Check sheet for the drawn part. Datum: minimum x, y, z corner. Units: mm. Coordinates: 2 decimals unless noted, no trailing zeros. Order: outer loops, then holes, each group sorted by start corner. A loop starts at its lowest first (then second) coordinate and runs counter-clockwise, first axis right, second up. Notation, with made-up numbers: (0.5, 41.5) -> (21.5, 41.5) arc R14 cw to (21.5, 47.5) -> close; hole circle Ø6 at (-14, -5). An arc over 180 degrees is marked (long way). Answer as CSV lines item,"result".
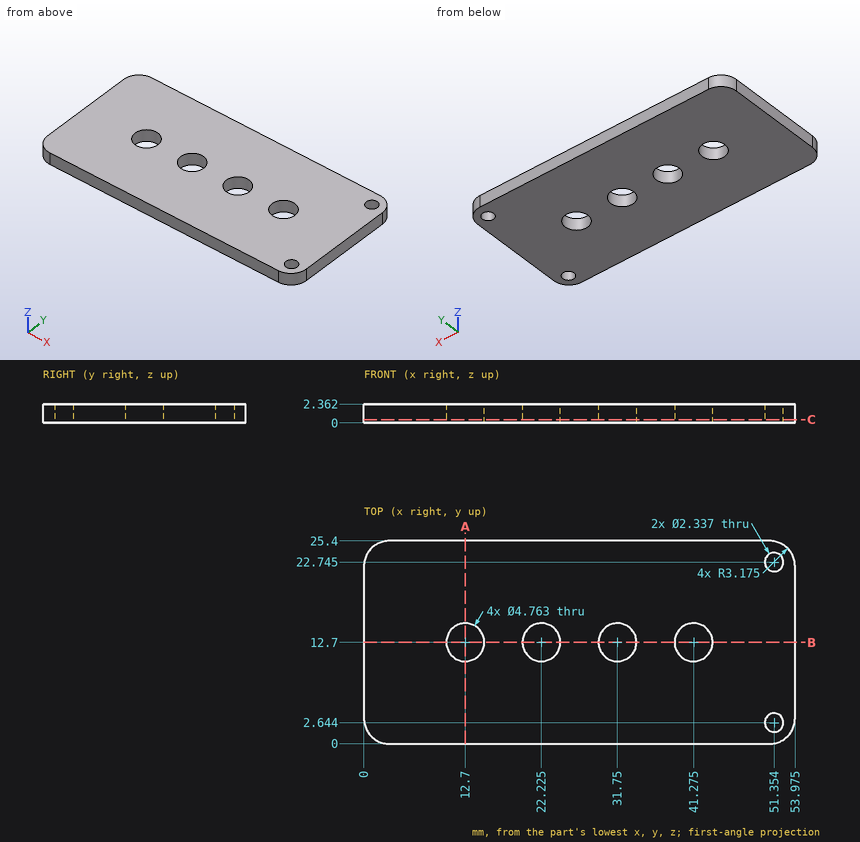
Item 1: Thickness scan on line 1 (Y direction, x = 31.75, z = 1.5); line 2 (X direction, y = 3.25, z = 1.9) (1 decimal); line 3 (Y direction, x = 30.5, z = 1.5) (1 decimal). Record the ranges inside material, lowest first.
Answer list:
line 1,"0 to 10.32, 15.08 to 25.4"
line 2,"0 to 50.4, 52.4 to 54"
line 3,"0 to 10.7, 14.7 to 25.4"
Item 2: Section check B-B, the plane y = 12.7. Record the boundary of the cut face in (x, z) (1 decimal).
Answer list:
outline,"(0, 0) -> (10.3, 0) -> (10.3, 2.4) -> (0, 2.4) -> close; (15.1, 0) -> (19.8, 0) -> (19.8, 2.4) -> (15.1, 2.4) -> close; (24.6, 0) -> (29.4, 0) -> (29.4, 2.4) -> (24.6, 2.4) -> close; (34.1, 0) -> (38.9, 0) -> (38.9, 2.4) -> (34.1, 2.4) -> close; (43.7, 0) -> (54, 0) -> (54, 2.4) -> (43.7, 2.4) -> close"
Item 3: Section check C-C, the plane z = 0.4. Count the separate pieces of the cut face and the enclosed holes in it, plus the area to 3 significant figures.
Answer list:
separate pieces,"1"
enclosed holes,"6"
area,"1,280 mm2"
Item 4: Section check A-A, the plane x = 12.7. Record the boundary of the cut face in (y, z).
Answer list:
outline,"(0, 0) -> (10.32, 0) -> (10.32, 2.36) -> (0, 2.36) -> close; (15.08, 0) -> (25.4, 0) -> (25.4, 2.36) -> (15.08, 2.36) -> close"
Item 5: Depth check by flat-ended pin: pin 1 Ø2 at (x, y) = (51.35, 2.64) entering from -Z. Enter the tip coordinate at first touch or a pass-through.
Answer list:
pin 1,"through"
